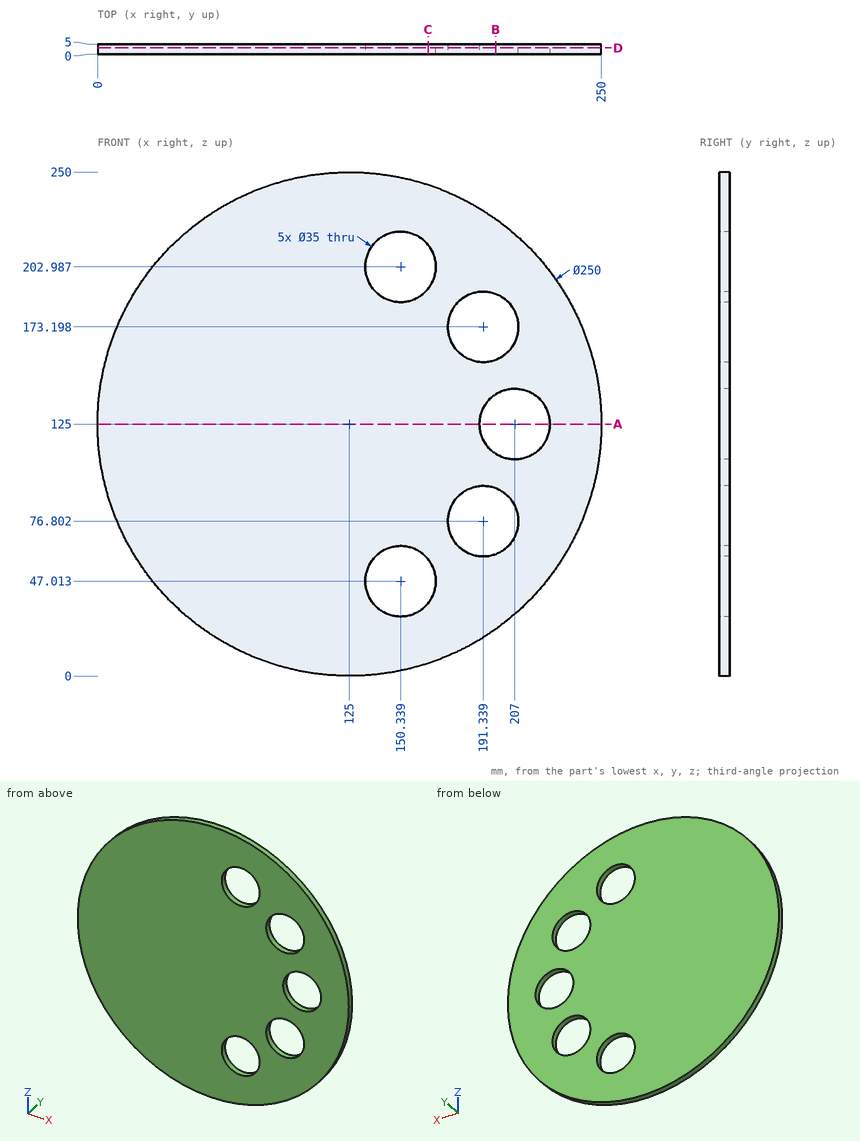
Can you work these out from the drawing? Everything is in mm from the part's minimum corner. Coordinates: 2 decimals unless noted, no trailing zeros. Loops run counter-clockwise (first coordinate to the right, second up) from the corner with the lowest first, then second, coordinate; pieces in that order, holes last.
1) Imagine slicing it at A-A (z = 125). List the corners of the cut face in (x, y) for me.
Reported:
outline: (0, 0) - (189.5, 0) - (189.5, 5) - (0, 5) - close; (224.5, 0) - (250, 0) - (250, 5) - (224.5, 5) - close
2) Please list where these lines run through material, in increasing order: line 1 along X through (y, z) = (3, 125); line 2 along Z through (x, y) = (166.5, 4.2) (1 decimal); line 3 along X through (y, z) = (3.95, 174) (1 decimal).
Reported:
line 1: x = 0 to 189.5, 224.5 to 250
line 2: z = 7.1 to 40.3, 53.7 to 196.3, 209.7 to 242.9
line 3: x = 10 to 173.9, 208.8 to 240
3) Imagine slicing it at D-D (y = 3.05). List the corners of the cut face in (x, z) for me, and give its area (3 significant figures).
Reported:
outline: circle Ø250 at (125, 125); hole circle Ø35 at (150.34, 47.01); hole circle Ø35 at (150.34, 202.99); hole circle Ø35 at (191.34, 76.8); hole circle Ø35 at (191.34, 173.2); hole circle Ø35 at (207, 125)
area: 44,300 mm2
4) Imagine slicing it at B-B (x = 197.5). List the corners of the cut face in (y, z) for me.
Reported:
outline: (0, 23.17) - (5, 23.17) - (5, 60.42) - (0, 60.42) - close; (0, 93.18) - (5, 93.18) - (5, 110.3) - (0, 110.3) - close; (0, 139.7) - (5, 139.7) - (5, 156.82) - (0, 156.82) - close; (0, 189.58) - (5, 189.58) - (5, 226.83) - (0, 226.83) - close
5) Will these pins go through, and if not, where does the flat tip stop? pin 1 Ø1.5 at (y, z) = (1, 166.5) entering from -X; pin 2 Ø3 at (x, y) = (47, 4) entering from -Z.
Reported:
pin 1: stops at x = 6.83
pin 2: stops at z = 26.14
6) Imagine slicing it at C-C (x = 164). List the corners of the cut face in (y, z) for me (1 decimal), and give its area (3 significant figures).
Reported:
outline: (0, 6.2) - (5, 6.2) - (5, 36.1) - (0, 36.1) - close; (0, 58) - (5, 58) - (5, 192) - (0, 192) - close; (0, 213.9) - (5, 213.9) - (5, 243.8) - (0, 243.8) - close
area: 969 mm2
